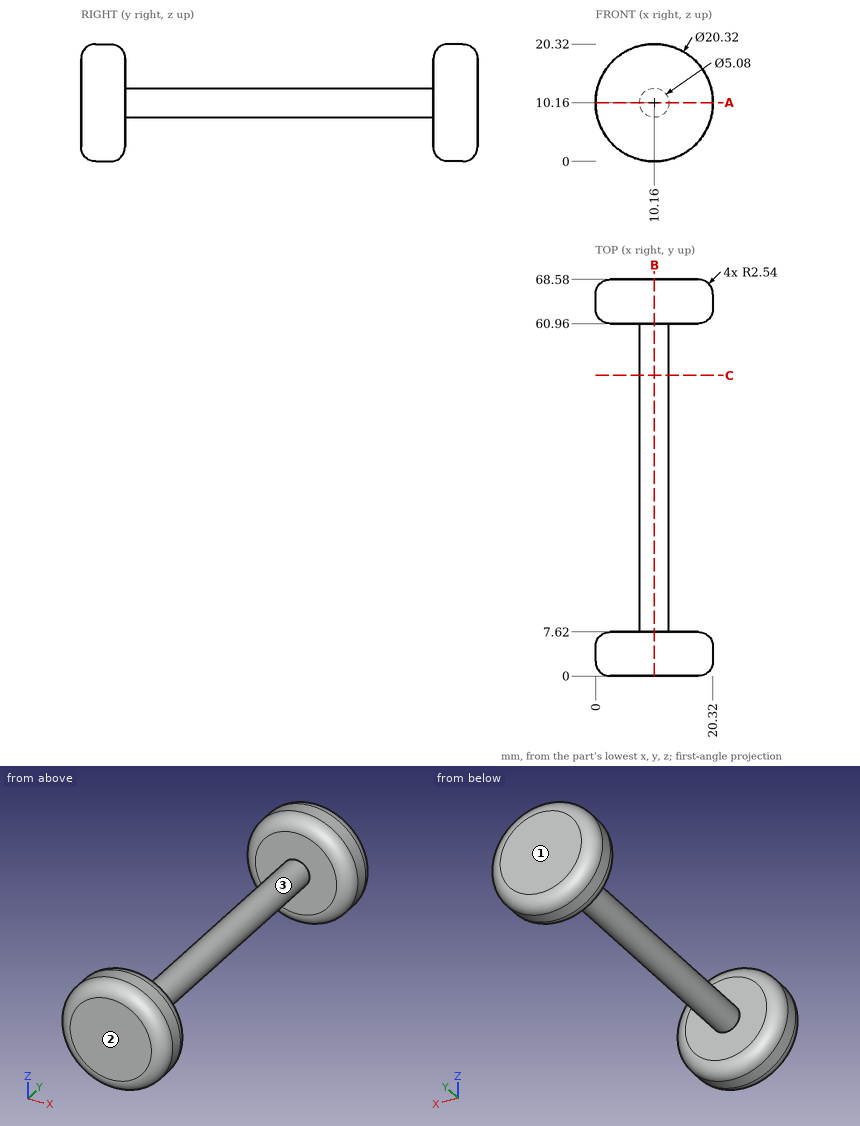
Geometry check sheet. Reference: drawing and pictorial views, mm from the part's lowest x, y, z. Coordinates: 2 decimals unless noted, no trailing zeros. Order: outer loops, then holes, each group sorted by start corner. A loop starts at its lowest first (then second) coordinate and runs counter-clockwise, first axis right, second up. Notation, with made-up numbers: (-38.5, -9) -> (9.5, -9) arc R16 ccw to (9.5, 11) -> close; hole circle Ø2 at (27.5, -14.5). An arc over 180 degrees is marked (long way). Use CSV: the item, a comma, the result in double quotes. Start each with the question number.
Q1. Section check A-A, the plane z = 10.16. Record the cut outline in (x, y).
Q2. Depth check by flat-ended pin: P1, Ø1, axis at x = 11.5, y = 31.5, coming from the +Z side; P2, Ø4, axis at y = 35, z = 16.5, coming from the -X side; P3, Ø12, axis at y = 40, z = 13, coming from the -X side. Enter the tip coordinate at first touch or a pass-through.
Q3. Section check B-B, the plane x = 10.16. Record the cut outline in (y, z).
Q4. Draft check along Y on the marked faces 1, 2 and 3. Enter one of: +Y half, -Y half, draft (parallel to the pull), parting line (faces both ways), or undercut.
Q5. Section check C-C, the plane y = 52. Record the cut outline in (x, z).
Q6. Thickness scan on line 1 along Y through (x, z) = (7.25, 11); line 2 along X through (y, z) = (52, 10.25); line 3 along Y through (x, z) = (19.25, 11.5). Record the ranges inside material, lowest first.
Returned:
1,outline,"(0, 2.54) arc R2.54 ccw to (2.54, 0) -> (17.78, 0) arc R2.54 ccw to (20.32, 2.54) -> (20.32, 5.08) arc R2.54 ccw to (17.78, 7.62) -> (12.7, 7.62) -> (12.7, 60.96) -> (17.78, 60.96) arc R2.54 ccw to (20.32, 63.5) -> (20.32, 66.04) arc R2.54 ccw to (17.78, 68.58) -> (2.54, 68.58) arc R2.54 ccw to (0, 66.04) -> (0, 63.5) arc R2.54 ccw to (2.54, 60.96) -> (7.62, 60.96) -> (7.62, 7.62) -> (2.54, 7.62) arc R2.54 ccw to (0, 5.08) -> close"
2,P1,"stops at z = 12.56"
2,P2,"passes through"
2,P3,"stops at x = 7.62"
3,outline,"(0, 2.54) arc R2.54 ccw to (2.54, 0) -> (5.08, 0) arc R2.54 ccw to (7.62, 2.54) -> (7.62, 7.62) -> (60.96, 7.62) -> (60.96, 2.54) arc R2.54 ccw to (63.5, 0) -> (66.04, 0) arc R2.54 ccw to (68.58, 2.54) -> (68.58, 17.78) arc R2.54 ccw to (66.04, 20.32) -> (63.5, 20.32) arc R2.54 ccw to (60.96, 17.78) -> (60.96, 12.7) -> (7.62, 12.7) -> (7.62, 17.78) arc R2.54 ccw to (5.08, 20.32) -> (2.54, 20.32) arc R2.54 ccw to (0, 17.78) -> close"
4,face 1,"+Y half"
4,face 2,"-Y half"
4,face 3,"undercut"
5,outline,"circle Ø5.08 at (10.16, 10.16)"
6,line 1,"y = 0 to 7.62, 60.96 to 68.58"
6,line 2,"x = 7.62 to 12.7"
6,line 3,"y = 0.54 to 7.08, 61.5 to 68.04"
